Design review of the part built by this model. Coordinates are the model's own, in mm. A direction names the side the tool comes from. Give positions to 0.01 mm unless a question says otherwise; leave off trailing zeros. Loops run counter-clockwise (first coordinate to the right, second up) from the corner with the lowest first, then second, coordinate; pieces in that order, holes last. Notation, with made-up numbers: M 0,42 L 18,42 A8 cw 18,46 Z; hole C 16.25,-10.75 d10. An arc over 180 degrees is marked long. Use a Markdown table: item, result. Add a question column.
(1) For probe 1 along X at (y, z) = (60.5, -479.5); probe 2 along X at (y, z) = (-345, -178); probe 3 along X at (y, z) = (222.5, -70), list the stretches that pass through material, from the lowest coordinate up.
(2) Add section C-C, the plane z = -693. Give the boundary of the cut face in (x, y), then the cut area to 3 significant figures.
(3) Draft analysis for pull direction X (two halves, no side actions). For faces 1 (the face through (-165.1, -293, -182)), 2 (the face through (-88.9, -279, -907)), 3 (the face through (736.2, 99.1, -232.1)), state which applies: pulls with the +X half, pulls with the -X half, needs draft (parallel to the pull), parting line crosses it, or undercut.
(4) Insertion check: pin 1 Ø4 at (x, z) = (691.5, -424) entering from -Y. The pin has a flat end and moves straight along its axis. Give the tip position at first contact, or say it passes through.
(5) For faces 4 (the face through (-63, 52, -266)), 5 (the face through (-63.14, -147.53, -653.21)), 6 (the face through (736.244, -153.798, -120.192)), list the 3-axis set-ups (+Z, -Z, +X, -X, +Y, -Y) from which the entire face can be reached by the end or side of a thin tool; tool diameter is ignored.
(6) Add section B-B, the plane y = -25.5. Give the boundary of the cut face in (x, z), then the cut area to 3 significant figures.
(7) Add section D-D, the plane x = 633.5. Give the boundary of the cut face in (y, z), then the cut area to 3 significant figures.
(8) Add section A-A, the plane z = -240.5. Give the boundary of the cut face in (x, y).
```python
from build123d import *

# Parameters (mm, degrees)
SKETCH1_W           = 673.1
SKETCH1_H           = 762
BOSS_EXTRUDE1_DEPTH = 254
SKETCH2_R           = 25.4
BOSS_EXTRUDE2_DEPTH = 38.1
BOSS_EXTRUDE3_DEPTH = 50.8
SKETCH4_R           = 127
BOSS_EXTRUDE4_DEPTH = 76.2


with BuildPart() as part:
    # Sketch1 → Boss-Extrude1 (new body)
    with BuildSketch(Plane(origin=(0, 0, 0), x_dir=(1, 0, 0), z_dir=(0, 1, 0))):
        with Locations((336.55, 381)):
            Rectangle(SKETCH1_W, SKETCH1_H)
    extrude(amount=BOSS_EXTRUDE1_DEPTH)

    # Sketch2 → Boss-Extrude2 (add)
    with BuildSketch(Plane(origin=(673.1, 0, 0), x_dir=(0, 0, -1), z_dir=(1, 0, 0))):
        with Locations((406.4, 88.9)):
            Circle(SKETCH2_R)
    boss_extrude2 = extrude(amount=BOSS_EXTRUDE2_DEPTH)

    # Sketch3 → Boss-Extrude3 (add)
    with BuildSketch(Plane(origin=(711.2, 0, 0), x_dir=(0, 0, -1), z_dir=(1, 0, 0))):
        with BuildLine():
            Line((422.726805286, 108.357528855), (925.855623983, -313.817677348))
            Line((925.855623983, -313.817677348), (909.528818697, -333.275206203))
            Line((909.528818697, -333.275206203), (893.202013411, -352.732735059))
            Line((893.202013411, -352.732735059), (406.4, 63.5))
            Line((406.4, 63.5), (121.876807164, 40.194732275))
            Line((121.876807164, 40.194732275), (217.686843741, -325.462787901))
            Line((217.686843741, -325.462787901), (193.116290848, -331.90079462))
            Line((193.116290848, -331.90079462), (168.545737954, -338.338801338))
            Line((168.545737954, -338.338801338), (70.465312804, 35.98362165))
            Line((70.465312804, 35.98362165), (66.845699755, 35.687139489))
            Line((66.845699755, 35.687139489), (64.804838024, 59.014295812))
            Line((64.804838024, 59.014295812), (62.591082159, 84.317641143))
            Line((62.591082159, 84.317641143), (406.4, 114.3))
            ThreePointArc((406.4, 114.3), (415.08731164, 112.768192568), (422.726805286, 108.357528855))
        make_face()
    boss_extrude3 = extrude(amount=BOSS_EXTRUDE3_DEPTH)

    # Sketch4 → Boss-Extrude4 (add)
    with BuildSketch(Plane(origin=(762, 0, 0), x_dir=(0, 0, -1), z_dir=(1, 0, 0))):
        with Locations((183.45928077, -295.044965279)):
            Circle(SKETCH4_R)
        with Locations((880.342525414, -308.784998274)):
            Circle(SKETCH4_R)
    boss_extrude4 = extrude(amount=BOSS_EXTRUDE4_DEPTH)

    # Mirror1: Boss-Extrude2, Boss-Extrude3, Boss-Extrude4 across plane
    add(boss_extrude2.mirror(Plane(origin=(336.55, 0, 0), x_dir=(0, 0, 1), z_dir=(1, 0, 0))))
    add(boss_extrude3.mirror(Plane(origin=(336.55, 0, 0), x_dir=(0, 0, 1), z_dir=(1, 0, 0))))
    add(boss_extrude4.mirror(Plane(origin=(336.55, 0, 0), x_dir=(0, 0, 1), z_dir=(1, 0, 0))))


solid = part.part
```
Established:
| question | item | result |
|---|---|---|
| 1 | probe 1 | -88.9 to -38.1, 0 to 673.1, 711.2 to 762 |
| 1 | probe 2 | -165.1 to -88.9, 762 to 838.2 |
| 1 | probe 3 | 0 to 673.1 |
| 2 | outline | M -88.9,-181.55 L -38.1,-181.55 L -38.1,-118.43 L -88.9,-118.43 Z; M 0,0 L 673.1,0 L 673.1,254 L 0,254 Z; M 711.2,-181.55 L 762,-181.55 L 762,-118.43 L 711.2,-118.43 Z |
| 2 | area | 177,000 mm^2 |
| 3 | face 1 | pulls with the -X half |
| 3 | face 2 | undercut |
| 3 | face 3 | needs draft |
| 4 | pin 1 | y = 68.86 |
| 5 | face 4 | -X |
| 5 | face 5 | -Y |
| 5 | face 6 | +Z, -Y |
| 6 | outline | M -88.9,-582.25 L -38.1,-582.25 L -38.1,-510.49 L -88.9,-510.49 Z; M -88.9,-139.09 L -38.1,-139.09 L -38.1,-86.58 L -88.9,-86.58 Z; M 711.2,-582.25 L 762,-582.25 L 762,-510.49 L 711.2,-510.49 Z; M 711.2,-139.09 L 762,-139.09 L 762,-86.58 L 711.2,-86.58 Z |
| 6 | area | 12,600 mm^2 |
| 7 | outline | M 0,-762 L 254,-762 L 254,0 L 0,0 Z |
| 7 | area | 194,000 mm^2 |
| 8 | outline | M -165.1,-408.51 L -88.9,-408.51 L -88.9,-181.58 L -165.1,-181.58 Z; M -88.9,49.91 L -38.1,49.91 L -38.1,99.83 L -88.9,99.83 Z; M 0,0 L 673.1,0 L 673.1,254 L 0,254 Z; M 711.2,49.91 L 762,49.91 L 762,99.83 L 711.2,99.83 Z; M 762,-408.51 L 838.2,-408.51 L 838.2,-181.58 L 762,-181.58 Z |
